The model under review builds one solid part; all positions refer to its coordinate system, in mm. A direction names the side the tool comes from. Round coordinates to 2 decimals unless told otherwise and drop trailing zeros. Write each loop counter-clockwise with the first axis right and the second up, starting at its lowest first coordinate (ties: lowest second). Pieces come first, ordered by that corner, then holes. Notation, with made-up numbers: (-0.5, 19.25) - (7.5, 19.25) arc R11 ccw to (7.5, 25.25) - close; hole circle Ø11 at (-10, 57). An arc over 180 degrees is marked (long way). Write each question's results on one line, items separated by ' | '.
```python
from build123d import *

# Parameters (mm, degrees)
F0_W     = 1000
F0_H     = 400
F1_DEPTH = 20
F2_W     = 20
F2_H     = 400
F3_DEPTH = 300
F4_R     = 5
F5_R     = 5
F6_R     = 5


with BuildPart() as f1:
    # F0 (on Top) → F1 (new body)
    with BuildSketch(Plane.XY):
        with Locations((-78.8800735027, -73.4630868891)):
            Rectangle(F0_W, F0_H)
    extrude(amount=F1_DEPTH)

    # F2 (on face) → F3 (join)
    with BuildSketch(Plane.XY):
        with Locations((-568.8800735027, -73.4630868891)):
            Rectangle(F2_W, F2_H)
        with Locations((411.1199264973, -73.4630868891)):
            Rectangle(F2_W, F2_H)
    extrude(amount=-F3_DEPTH)

    # F4
    f4_edges = [f1.edges().sort_by_distance(p)[0] for p in [
        (-78.880074, -273.463087, 20),
    ]]
    fillet(f4_edges, radius=F4_R)

    # F5
    f5_edges = [f1.edges().sort_by_distance(p)[0] for p in [
        (421.119926, -70.963087, 20),
    ]]
    fillet(f5_edges, radius=F5_R)

    # F6
    f6_edges = [f1.edges().sort_by_distance(p)[0] for p in [
        (401.119926, -273.463087, -150),
        (-578.880074, -70.963087, 20),
    ]]
    fillet(f6_edges, radius=F6_R)


solid = f1.part
```
Q1. Tool access review of faces 1 (the flat face through (-229, 126.537, 3)), 2 (the flat face through (401.12, -74, -148)): name each direction out of +Z, -Z, +X, -X, +Y, -Y from which nothing blocks a thin tool from reaching the whole face with its end or side.
Evaluation:
face 1: +Z, -Z, +X, -X, +Y | face 2: -Z, +Y, -Y
Q2. The part is to be moulded in two halves that separate along X. For faces 3 (the flat face through (-578.88, -74, -140)), 4 (the flat face through (-81, -273.463, 10)), 5 (the flat face through (-83, -71, 0)), say which applies: released by +X, released by -X, zero draft, split by the parting line, or undercut.
Evaluation:
face 3: released by -X | face 4: zero draft | face 5: undercut
Q3. For probe 1 along X at (y, z) = (31.5, -107); probe 2 along Z at (x, y) = (-143, 55), list the stretches that pass through material, from the lowest coordinate up.
Evaluation:
probe 1: x = -578.88 to -558.88, 401.12 to 421.12 | probe 2: z = 0 to 20
Q4. We need section C-C (x = -503). State the section outline as (y, z) points.
Evaluation:
outline: (-273.46, 0) - (126.54, 0) - (126.54, 20) - (-268.46, 20) arc R5 ccw to (-273.46, 15) - close
Q5. We need section B-B (y = -17.5). State the section outline as (x, z) points, plus the area to 3 significant figures.
Evaluation:
outline: (-578.88, -300) - (-558.88, -300) - (-558.88, 0) - (401.12, 0) - (401.12, -300) - (421.12, -300) - (421.12, 15) arc R5 ccw to (416.12, 20) - (-573.88, 20) arc R5 ccw to (-578.88, 15) - close | area: 32,000 mm^2
Q6. We need section A-A (z = -92.5). State the section outline as (x, y) points.
Evaluation:
outline: (-578.88, -268.46) arc R5 ccw to (-573.88, -273.46) - (-558.88, -273.46) - (-558.88, 126.54) - (-578.88, 126.54) - close; (401.12, -268.46) arc R5 ccw to (406.12, -273.46) - (416.12, -273.46) arc R5 ccw to (421.12, -268.46) - (421.12, 126.54) - (401.12, 126.54) - close
Q7. Insertion check: P1, Ø10, axis at x = -375.5, y = -65.5, coming from the -Z side. The pin has a flat end and moves straight along its axis. Give the tip position at first contact, or say it passes through.
Evaluation:
P1: stops at z = 0
